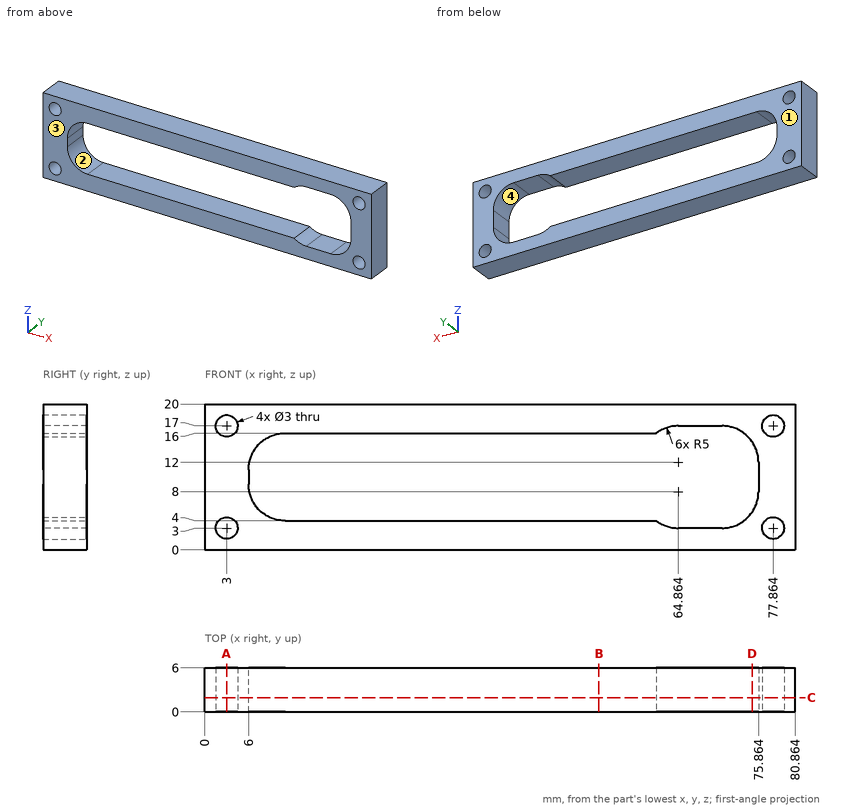
Study the drawing (mm; zero at the part's minimum x, y, z) and answer. A direction names the side the tool comes from. Coordinates: 2 decimals unless noted, no trailing zeros. Loops run counter-clockwise (first coordinate to the right, second up) from the corner with the lowest first, then second, coordinate; pieces in that order, holes last. Notation, with made-up numbers: (32, 62) -> (75, 62) arc R33 ccw to (75, 93) -> close; hole circle Ø7 at (59, 51). An arc over 180 degrees is marked (long way). Write item = value, one per line. Start each with the question number.
1) The mould has two halves that part along X. Classify the marked faces 1 and 2: pulls with the +X half, pulls with the -X half, needs draft (parallel to the pull), parting line crosses it, or undercut.
2) The part is cut by section A-A, the plane x = 3. Determine the outline of the cut face in (y, z).
3) Find the intervals of material crossed by L1, parallel to Z at x = 36.5, y = 2.5; L2, parallel to Z at x = 65.5, y = 1.8; L3, parallel to X at y = 3.45, z = 17.5, in increasing order. Write a range as from..to.
4) For the marked faces 3 and 4, determine the directions among +Z, -Z, +X, -X, +Y, -Y from which every point of the face is accessible in a straight line to the end or side of a thin tool.
5) The part is cut by section D-D, the plane x = 75. Determine the outline of the cut face in (y, z).
6) The part is cut by section C-C, the plane y = 1.95. Determine the outline of the cut face in (x, z).
7) The part is cut by section B-B, the plane x = 54. Determine the outline of the cut face in (y, z), plus the area to 3 significant figures.
Result:
q1.face_1 = needs draft
q1.face_2 = undercut
q2.outline = (0, 0) -> (6, 0) -> (6, 1.5) -> (0, 1.5) -> close; (0, 4.5) -> (6, 4.5) -> (6, 15.5) -> (0, 15.5) -> close; (0, 18.5) -> (6, 18.5) -> (6, 20) -> (0, 20) -> close
q3.L1 = 0..4, 16..20
q3.L2 = 0..3, 17..20
q3.L3 = 0..1.59, 4.41..76.45, 79.28..80.86
q4.face_3 = +Z, -Z, +X, -X, -Y
q4.face_4 = +Y, -Y
q5.outline = (0, 0) -> (6, 0) -> (6, 5.19) -> (0, 5.19) -> close; (0, 14.81) -> (6, 14.81) -> (6, 20) -> (0, 20) -> close
q6.outline = (0, 0) -> (80.86, 0) -> (80.86, 20) -> (0, 20) -> close; hole circle Ø3 at (3, 3); hole circle Ø3 at (3, 17); hole (6, 9) arc R5 ccw to (11, 4) -> (61.86, 4) arc R5 ccw to (64.86, 3) -> (70.86, 3) arc R5 ccw to (75.86, 8) -> (75.86, 12) arc R5 ccw to (70.86, 17) -> (64.86, 17) arc R5 ccw to (61.86, 16) -> (11, 16) arc R5 ccw to (6, 11) -> close; hole circle Ø3 at (77.86, 3); hole circle Ø3 at (77.86, 17)
q7.outline = (0, 0) -> (6, 0) -> (6, 4) -> (0, 4) -> close; (0, 16) -> (6, 16) -> (6, 20) -> (0, 20) -> close
q7.area = 48.0 mm²
